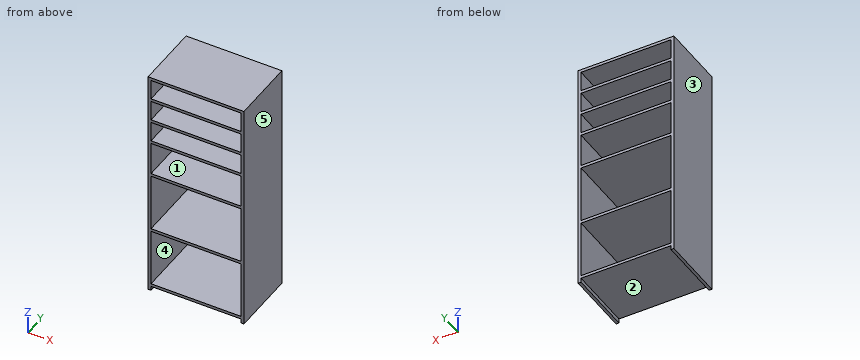
```python
from build123d import *

# Parameters (mm, degrees)
F0_W     = 620
F0_H     = 400
F0_H_2   = 230
F0_H_3   = 140
F1_DEPTH = 450


with BuildPart() as f1:
    # F0 (on Front) → F1 (new body)
    with BuildSketch(Plane.XZ):
        Polygon((0, 1620), (0, 0), (20, 0), (20, 30), (640, 30), (640, 0), (660, 0), (660, 1620), align=None)
        with Locations((330, 250)):
            Rectangle(F0_W, F0_H, mode=Mode.SUBTRACT)
        with Locations((330, 670)):
            Rectangle(F0_W, F0_H, mode=Mode.SUBTRACT)
        with Locations((330, 1005)):
            Rectangle(F0_W, F0_H_2, mode=Mode.SUBTRACT)
        with Locations((330, 1210)):
            Rectangle(F0_W, F0_H_3, mode=Mode.SUBTRACT)
        with Locations((330, 1370)):
            Rectangle(F0_W, F0_H_3, mode=Mode.SUBTRACT)
        with Locations((330, 1530)):
            Rectangle(F0_W, F0_H_3, mode=Mode.SUBTRACT)
    extrude(amount=F1_DEPTH)


solid = f1.part
```
Check sheet for the modelled part. Datum: model origin and axes. Units: mm. Face numbers are marked on the shaded views. A direction names the side the tool comes from. Give positions to 0.01 mm unless a question says otherwise; leave off trailing zeros. Loops run counter-clockwise (first coordinate to the right, second up) from the corner with the lowest first, then second, coordinate; pieces in that order, holes last. Notation, with made-up numbers: M 59.5,3.25 L 89.5,3.25 A23 ccw 89.5,32.25 Z; hole C 22.5,87 d1. An arc over 180 degrees is marked long. Answer in a Markdown table with one row per item.
1) Depth check by flat-ended pin: pin 1 (3 mm diameter, centred on x = 177.5, y = -148.5, fed in from -Z). Enter the tip coordinate at first touch or a pass-through.
Solutions:
| item | result |
|---|---|
| pin 1 | stops at z = 30 |
2) Cross-section at C-C (y = -389.5). Count the separate pieces of the cut face and the enclosed holes in it, plus the area to 3 significant figures.
Solutions:
| item | result |
|---|---|
| separate pieces | 1 |
| enclosed holes | 6 |
| area | 152,000 mm^2 |
3) Mould release check, pull along X, two halves, no side actions. Record for the marked faces 3, 4 and 5: released by +X, released by -X, zero draft, split by the parting line, or undercut.
Solutions:
| item | result |
|---|---|
| face 3 | released by -X |
| face 4 | undercut |
| face 5 | released by +X |
4) Thickness scan on line 1 (X direction, y = -362.5, z = 959). Record the ranges inside material, lowest first.
Solutions:
| item | result |
|---|---|
| line 1 | x = 0 to 20, 640 to 660 |
5) Cross-section at B-B (z = 373.5). Enter the section's corners in (x, y), plus the area to 3 significant figures.
Solutions:
| item | result |
|---|---|
| outline | M 0,-450 L 20,-450 L 20,0 L 0,0 Z; M 640,-450 L 660,-450 L 660,0 L 640,0 Z |
| area | 18,000 mm^2 |
6) Cross-section at A-A (x = 410.5). Enter the section's corners in (y, z).
Solutions:
| item | result |
|---|---|
| outline | M -450,30 L 0,30 L 0,50 L -450,50 Z; M -450,450 L 0,450 L 0,470 L -450,470 Z; M -450,870 L 0,870 L 0,890 L -450,890 Z; M -450,1120 L 0,1120 L 0,1140 L -450,1140 Z; M -450,1280 L 0,1280 L 0,1300 L -450,1300 Z; M -450,1440 L 0,1440 L 0,1460 L -450,1460 Z; M -450,1600 L 0,1600 L 0,1620 L -450,1620 Z |
7) Tool access check on the marked faces 1 and 2. Record the directions out of +Z, -Z, +X, -X, +Y, -Y that give a thin tool (end or side, any length) a straight path to the whole face; none if there is none.
Solutions:
| item | result |
|---|---|
| face 1 | +Y, -Y |
| face 2 | -Z, +Y, -Y |
